from build123d import *

# Parameters (mm, degrees)
BOSS_EXTRUDE1_DEPTH = 38.1
SKETCH2_R           = 2
CUT_EXTRUDE1_DEPTH  = 52.38473752


with BuildPart() as part:
    # Sketch1 → Boss-Extrude1 (new body)
    with BuildSketch(Plane(origin=(0, 0, 0), x_dir=(1, 0, 0), z_dir=(0, 1, 0))):
        with BuildLine():
            Line((3, 15.875), (3, 23.875))
            Line((3, 23.875), (6, 23.875))
            Line((6, 23.875), (6, 17.895966724))
            ThreePointArc((6, 17.895966724), (0, -18.875), (-6, 17.895966724))
            Line((-6, 17.895966724), (-6, 23.875))
            Line((-6, 23.875), (-3, 23.875))
            Line((-3, 23.875), (-3, 15.875))
            Line((-3, 15.875), (-3, 15.588958432))
            ThreePointArc((-3, 15.588958432), (0, -15.875), (3, 15.588958432))
            Line((3, 15.588958432), (3, 15.875))
        make_face()
    extrude(amount=BOSS_EXTRUDE1_DEPTH)

    # Sketch2 → Cut-Extrude1 (cut, through all)
    with BuildSketch(Plane.ZY.offset(6)):
        with Locations((-20.885483362, 33.1)):
            Circle(SKETCH2_R)
        with Locations((-20.885483362, 5)):
            Circle(SKETCH2_R)
    extrude(amount=-CUT_EXTRUDE1_DEPTH, mode=Mode.SUBTRACT)


solid = part.part
Geometry check sheet. Reference: the model listing, model coordinates, mm. A direction names the side the tool comes from. Give positions to 0.01 mm unless a question says otherwise; leave off trailing zeros. Order: outer loops, then holes, each group sorted by start corner. A loop starts at its lowest first (then second) coordinate and runs counter-clockwise, first axis right, second up. Notation, with made-up numbers: (-40, 70.5) - (-28, 70.5) arc R21 ccw to (-28, 75.5) - close; hole circle Ø3 at (-26.5, 14). An arc over 180 degrees is marked (long way). Answer as a JSON object with one key per item and string values.
(1) Material ranges on line 1 (X direction, y = 28, z = 0) (3 decimals); line 2 (X direction, y = 16.5, z = -20.5); line 3 (Z direction, x = -0.5, y = 7), recorded low to high.
Report:
{"line 1": "-18.875 to -15.875, 15.875 to 18.875", "line 2": "-6 to -3, 3 to 6", "line 3": "15.87 to 18.87"}
(2) Cross-section at C-C (x = -8). Record the cut outline in (y, z).
Report:
{"outline": "(0, -17.1) - (38.1, -17.1) - (38.1, -13.71) - (0, -13.71) - close; (0, 13.71) - (38.1, 13.71) - (38.1, 17.1) - (0, 17.1) - close"}
(3) Cross-section at A-A (z = 0). Record the cut outline in (x, y) (3 decimals), then the cut area to 3 significant figures.
Report:
{"outline": "(-18.875, 0) - (-15.875, 0) - (-15.875, 38.1) - (-18.875, 38.1) - close; (15.875, 0) - (18.875, 0) - (18.875, 38.1) - (15.875, 38.1) - close", "area": "229 mm^2"}
(4) Draft check along Z on faces 4 (the cylindrical face through (-0.66, 18.78, 15.86)), 5 (the flat face through (4, 19, -23.875)), 6 (the flat face through (8, 38.1, -14)). Enter one of: released by +Z, released by -Z, zero draft, split by the parting line, or undercut.
Report:
{"face 4": "undercut", "face 5": "released by -Z", "face 6": "zero draft"}
(5) Tool access check on faces 1 (the flat face through (-3, 19, -20)), 2 (the flat face through (6, 19, -21)), 3 (the flat face through (-6, 19, -21)). Record the directions out of +Z, -Z, +X, -X, +Y, -Y that give a thin tool (end or side, any length) a straight path to the whole face; none if there is none.
Report:
{"face 1": "-Z, +Y, -Y", "face 2": "-Z, +X, +Y, -Y", "face 3": "-Z, -X, +Y, -Y"}
(6) Cross-section at D-D (y = 30.5). Record the cut outline in (x, z) (3 decimals).
Report:
{"outline": "(-6, -23.875) - (-3, -23.875) - (-3, -15.589) arc R15.875 cw (long way) to (3, -15.589) - (3, -23.875) - (6, -23.875) - (6, -17.896) arc R18.875 ccw (long way) to (-6, -17.896) - close"}
(7) Cross-section at B-B (y = 5). Record the cut outline in (x, z) (3 decimals).
Report:
{"outline": "(-6, -23.875) - (-3, -23.875) - (-3, -22.885) - (-6, -22.885) - close; (-6, -18.885) - (-3, -18.885) - (-3, -15.589) arc R15.875 cw (long way) to (3, -15.589) - (3, -18.885) - (6, -18.885) - (6, -17.896) arc R18.875 ccw (long way) to (-6, -17.896) - close; (3, -23.875) - (6, -23.875) - (6, -22.885) - (3, -22.885) - close"}
(8) Depth check by flat-ended pin: pin 1 Ø5 at (y, z) = (5, -20.89) entering from +X; pin 2 Ø4.5 at (y, z) = (5, -20.89) entering from -X; pin 3 Ø5 at (x, y) = (6, 15) entering from +Z. Enter the tip coordinate at first touch or a pass-through.
Report:
{"pin 1": "x = 6", "pin 2": "x = -6", "pin 3": "z = 18.55"}
